Design review of the part built by this model. Coordinates are the model's own, in mm. A direction names the side the tool comes from. Coordinates: 2 decimals unless noted, no trailing zeros. Loops run counter-clockwise (first coordinate to the right, second up) from the corner with the lowest first, then second, coordinate; pieces in that order, holes last. Notation, with made-up numbers: (4, -39.75) - (48, -39.75) arc R25 cw to (48, -17.75) - close; hole circle Ø10 at (-23.75, 70). An arc over 180 degrees is marked (long way). Answer in a Markdown table with one row per item. Add a question column.
(1) Clearance check with flat-ended pins moving along their axes: pin 1 (3 mm diameter, centred on x = 4, y = -3.5, fed in from -Z); pin 2 (3 mm diameter, centred on y = 6, z = -2, fed in from -X); pin 3 (1.5 mm diameter, centred on y = 6, z = 5, fed in from -X). State where each tip first meets the part, or that it passes through.
(2) We need section B-B, the plane x = 0. Write out the cut boundary in (y, z) (3 decimals).
(3) We need section A-A, the plane y = 0. Write out the cut boundary in (x, z) (3 decimals), plus the area to 3 significant figures.
(4) The part is to be moulded in two halves that separate along Y. For faces 4 (the face through (-0.217, -0.976, 11.557)), 5 (the face through (-6.37, -4.88, 5.94)), 6 (the face through (0, 5, -5)), say which applies: released by +Y, released by -Y, zero draft, split by the parting line, or undercut.
(5) We need section D-D, the plane z = 3.5. Write out the cut boundary in (x, y) (3 decimals), plus the area to 3 significant figures.
(6) To check wall thickness, follow L1, parallel to Y at x = 0, z = 11.3 (3 decimals); L2, parallel to Z at x = -3.5, y = 4.5; L3, parallel to Y at x = 1.5, z = 8. State the ranges of each line that lie inside material, in increasing order. Write a range as [from, to].
(7) We need section C-C, the plane z = -0.5. Write out the cut boundary in (x, y).
(8) For faces 1 (the face through (-0.065, 4.504, -2.465)), 2 (the face through (0, 0, 11.05)), 3 (the face through (0, -5, -5)), list the 3-axis set-ups (+Z, -Z, +X, -X, +Y, -Y) from which the entire face can be reached by the end or side of a thin tool; tool diameter is ignored.
from build123d import *

# Parameters (mm, degrees)
CYLINDER_R     = 8.025
CYLINDER_DEPTH = 12.05
SKETCH_R       = 0.5
PAD_DEPTH      = 5
SKETCH001_R    = 1
POCKET_DEPTH   = 1


with BuildPart() as part:
    # Cylinder → Cylinder (new body)
    with BuildSketch(Plane.XY):
        Circle(CYLINDER_R)
    extrude(amount=CYLINDER_DEPTH)

    # Sketch → Pad (new body)
    with BuildSketch(Plane(origin=(0, 0, 0), x_dir=(1, 0, 0), z_dir=(0, 0, -1))):
        with Locations((0, 5)):
            Circle(SKETCH_R)
        with Locations((0, -5)):
            Circle(SKETCH_R)
    extrude(amount=PAD_DEPTH)

    # Sketch001 → Pocket (cut)
    with BuildSketch(Plane.XY.offset(12.05)):
        Circle(SKETCH001_R)
    extrude(amount=-POCKET_DEPTH, mode=Mode.SUBTRACT)


solid = part.part
Responses:
| question | item | result |
|---|---|---|
| 1 | pin 1 | stops at z = 0 |
| 1 | pin 2 | stops at x = -0.5 |
| 1 | pin 3 | stops at x = -6.07 |
| 2 | outline | (-8.025, 0) - (-5.5, 0) - (-5.5, -5) - (-4.5, -5) - (-4.5, 0) - (4.5, 0) - (4.5, -5) - (5.5, -5) - (5.5, 0) - (8.025, 0) - (8.025, 12.05) - (1, 12.05) - (1, 11.05) - (-1, 11.05) - (-1, 12.05) - (-8.025, 12.05) - close |
| 3 | outline | (-8.025, 0) - (8.025, 0) - (8.025, 12.05) - (1, 12.05) - (1, 11.05) - (-1, 11.05) - (-1, 12.05) - (-8.025, 12.05) - close |
| 3 | area | 191 mm2 |
| 4 | face 4 | undercut |
| 4 | face 5 | split by the parting line |
| 4 | face 6 | zero draft |
| 5 | outline | circle Ø16.05 at (0, 0) |
| 5 | area | 202 mm2 |
| 6 | L1 | y = [-8.025, -1], [1, 8.025] |
| 6 | L2 | z = [0, 12.05] |
| 6 | L3 | y = [-7.88, 7.88] |
| 7 | outline | circle Ø1 at (0, -5); circle Ø1 at (0, 5) |
| 8 | face 1 | -Z |
| 8 | face 2 | +Z |
| 8 | face 3 | -Z, +X, -X, +Y, -Y |
